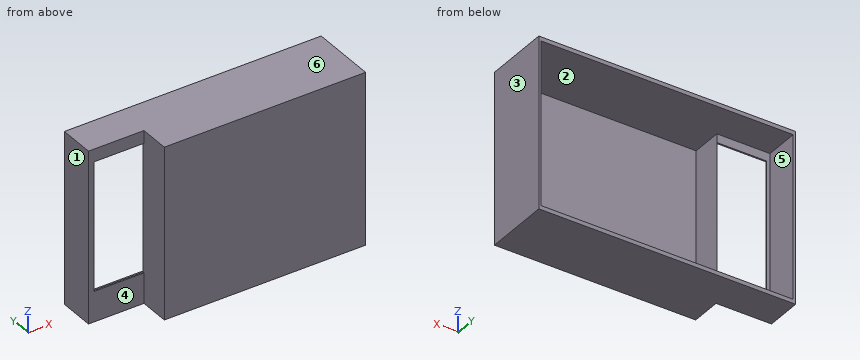
from build123d import *

# Parameters (mm, degrees)
F0_W     = 27.51
F0_H     = 16.75
F0_H_2   = 7
F1_DEPTH = 36.4
F3_DEPTH = 94.9
F4_W     = 139.175252
F4_H     = 90.411716
F4_W_2   = 27.51
F4_H_2   = 71.15
F5_DEPTH = 19
F6_W     = 109.82249
F6_H     = 90.411716
F7_DEPTH = 17


with BuildPart() as f1:
    # F0 (on Front) → F1 (new body)
    with BuildSketch(Plane.XZ):
        Polygon((-40.275, -47.45), (70.925, -47.45), (70.925, 47.45), (-40.275, 47.45), (-40.275, 40.45), (-40.275, -30.7), align=None)
        with Locations((-54.03, -39.075)):
            Rectangle(F0_W, F0_H)
        Polygon((-70.925, -47.45), (-67.785, -47.45), (-67.785, -30.7), (-67.785, 40.45), (-67.785, 47.45), (-70.925, 47.45), align=None)
        with Locations((-54.03, 43.95)):
            Rectangle(F0_W, F0_H_2)
    extrude(amount=F1_DEPTH)

    # F2 (on face) → F3 (cut)
    with BuildSketch(Plane(origin=(0, 0, -47.45), x_dir=(1, 0, 0), z_dir=(0, 0, -1))):
        Polygon((-40.275, 36.4), (-65.575, 36.4), (-70.925, 36.4), (-70.925, 19.75), (-40.275, 19.75), align=None)
    extrude(amount=-F3_DEPTH, mode=Mode.SUBTRACT)

    # F4 (on face) → F5 (cut)
    with BuildSketch(Plane(origin=(0, 0, 0), x_dir=(-1, 0, 0), z_dir=(0, 1, 0))):
        Rectangle(F4_W, F4_H)
        with Locations((54.03, 4.875)):
            Rectangle(F4_W_2, F4_H_2, mode=Mode.SUBTRACT)
    extrude(amount=-F5_DEPTH, mode=Mode.SUBTRACT)

    # F6 (on face) → F7 (cut)
    with BuildSketch(Plane(origin=(0, -19, 0), x_dir=(-1, 0, 0), z_dir=(0, 1, 0))):
        with Locations((-14.676381, 0)):
            Rectangle(F6_W, F6_H)
    extrude(amount=-F7_DEPTH, mode=Mode.SUBTRACT)


solid = f1.part
Input: part model. Units: mm. Frame: model coordinates. Face numbers are marked on the shaded views. A direction names the side the tool comes from. Coordinates: 2 decimals unless noted, no trailing zeros. Loops run counter-clockwise (first coordinate to the right, second up) from the corner with the lowest first, then second, coordinate; pieces in that order, holes last. Notation, with made-up numbers: (70, -16.5) -> (113, -16.5) arc R24 cw to (113, 19.5) -> close; hole circle Ø5 at (63.25, 58). An arc over 180 degrees is marked (long way). One line per item, written item: value.
(1) Cut plane D-D (z = -38). Output: boundary loops of the cut face in (x, y) (3 decimals), then the cut area to 3 significant figures.
Answer below:
outline: (-70.925, -19.75) -> (-40.275, -19.75) -> (-40.275, -36.4) -> (70.925, -36.4) -> (70.925, 0) -> (69.588, 0) -> (69.588, -36) -> (-40.235, -36) -> (-40.235, -19) -> (-69.588, -19) -> (-69.588, 0) -> (-70.925, 0) -> close
area: 142 mm2
(2) Draft query along X for the marked faces 1, 2 and 3. Return one class per face: pulls with the +X half, pulls with the -X half, needs draft (parallel to the pull), parting line crosses it, or undercut.
Answer below:
face 1: pulls with the -X half
face 2: undercut
face 3: pulls with the +X half
(3) Cut plane A-A (z = 14). Output: boundary loops of the cut face in (x, y) (3 decimals).
Answer below:
outline: (-70.925, -19.75) -> (-67.785, -19.75) -> (-67.785, -19) -> (-69.588, -19) -> (-69.588, 0) -> (-70.925, 0) -> close; (-40.275, -36.4) -> (70.925, -36.4) -> (70.925, 0) -> (69.588, 0) -> (69.588, -36) -> (-40.235, -36) -> (-40.235, -19) -> (-40.275, -19) -> close
(4) Set-up query: the marked faces 4, 5 and 6. Return all of +Z, -Z, +X, -X, +Y, -Y with unobstructed straight access to the full face (end or side cutting, diameter ignored); none if empty.
Answer below:
face 4: +Z, -Z, -X, -Y
face 5: +Y
face 6: +Z, +X, -X, +Y, -Y
(5) Ray query, line 1 along X through (y, z) = (-3.5, -41.5) (3 decimals); line 2 along Z through (x, y) = (31.5, -6.5); line 3 along Y through (x, z) = (45, 16.5). Return the intervals inside material, ascending.
Answer below:
line 1: x = -70.925 to -69.588, 69.588 to 70.925
line 2: z = -47.45 to -45.21, 45.21 to 47.45
line 3: y = -36.4 to -36
(6) Cut plane C-C (x = 43.5). Output: boundary loops of the cut face in (y, z), then the cut area to 3 significant figures.
Answer below:
outline: (-36.4, -47.45) -> (0, -47.45) -> (0, -45.21) -> (-36, -45.21) -> (-36, 45.21) -> (0, 45.21) -> (0, 47.45) -> (-36.4, 47.45) -> close
area: 200 mm2
(7) Cut plane B-B (y = -13). Output: boundary loops of the cut face in (x, z) (3 decimals).
Answer below:
outline: (-70.925, -47.45) -> (70.925, -47.45) -> (70.925, 47.45) -> (-70.925, 47.45) -> close; hole (-69.588, -45.206) -> (69.588, -45.206) -> (69.588, 45.206) -> (-69.588, 45.206) -> close
(8) Pin query (flat end, axial travel): pin 1 Ø19 at (y, z) = (-30.5, 4.5) entering from -X (3 decimals). Return the tip coordinate at first contact, or that it passes through.
Answer below:
pin 1: stops at x = -40.275
